Geometry check sheet. Reference: the model listing, model coordinates, mm. A direction names the side the tool comes from. Coordinates: 2 decimals unless noted, no trailing zeros. Write each loop counter-clockwise with the first axis right and the second up, starting at its lowest first coordinate (ties: lowest second). Pieces come first, ordered by that corner, then holes. Notation, with made-up numbers: (23.5, 49) -> (44.5, 49) arc R31 ccw to (44.5, 79) -> close; hole circle Ø8 at (52.25, -7). An arc over 180 degrees is marked (long way). Answer in a Markdown table with one row per item. Add a question column.
1. Cross-section at D-D on z = -3.81. Record the cut outline in (x, y).
2. Mould release check, pull along Z, two halves, no side actions. Record for faces 1 (the flat face through (4, 0, -73)), 2 (the flat face through (0, 2, -71)), 3 (the flat face through (63, 2, -143.764)): pulls with the +Z half, pulls with the -Z half, needs draft (parallel to the pull), parting line crosses it, or undercut.
3. Cross-section at C-C on x = 124.46. Record the cut outline in (y, z).
4. Scan lines: L1, parallel to X at y = 1.7, z = -3.81; L2, parallel to X at y = 1.5, z = -124; L3, parallel to X at y = 2.05, z = -139. Record each from-to range of solid material in increasing order. Write a range as from..to.
5. Set-up check for faces 4 (the flat face through (63, 2, 0)), 5 (the flat face through (63, 2, -128.524)), 6 (the flat face through (128.27, 2, -71)): record each of +Z, -Z, +X, -X, +Y, -Y from which the full face is reachable in a straight line by a thin tool's end or side.
6. Cross-section at A-A on z = -94.5. Record the cut outline in (x, y).
7. Cross-section at B-B on x = 20.5. Record the cut outline in (y, z).
8. Depth check by flat-ended pin: P1, Ø5, axis at x = 124.46, z = -139.954, coming from the -Y side; P2, Ø0.9, axis at x = 40.5, y = 1, coming from the -Z side; P3, Ø1.5, axis at y = 1, z = -45, coming from the +X side; P4, Ø0.9, axis at y = 2, z = -66, coming from the -X side. Enter the tip coordinate at first touch or a pass-through.
```python
from build123d import *

# Parameters (mm, degrees)
SKETCH1_W           = 128.27
SKETCH1_H           = 143.764
SKETCH1_W_2         = 97.79
SKETCH1_H_2         = 113.284
BOSS_EXTRUDE1_DEPTH = 3.048
SKETCH2_R           = 2.794
CUT_EXTRUDE1_DEPTH  = 3.302
SKETCH4_R           = 5.842
SKETCH4_R_2         = 2.794
BOSS_EXTRUDE2_DEPTH = 3.048


with BuildPart() as part:
    # Sketch1 → Boss-Extrude1 (new body)
    with BuildSketch(Plane(origin=(0, 0, 0), x_dir=(1, 0, 0), z_dir=(0, 1, 0))):
        with Locations((64.135, 71.882)):
            Rectangle(SKETCH1_W, SKETCH1_H)
        with Locations((64.135, 71.882)):
            Rectangle(SKETCH1_W_2, SKETCH1_H_2, mode=Mode.SUBTRACT)
    extrude(amount=BOSS_EXTRUDE1_DEPTH)

    # Sketch2 → Cut-Extrude1 (cut)
    with BuildSketch(Plane(origin=(0, 3.048, 0), x_dir=(1, 0, 0), z_dir=(0, 1, 0))):
        with Locations(Location((3.81, 139.954, 0), (0, 0, 270))):
            Circle(SKETCH2_R)
        with Locations(Location((124.46, 139.954, 0), (0, 0, 270))):
            Circle(SKETCH2_R)
        with Locations(Location((124.46, 3.81, 0), (0, 0, 270))):
            Circle(SKETCH2_R)
        with Locations(Location((3.81, 3.81, 0), (0, 0, 270))):
            Circle(SKETCH2_R)
    extrude(amount=-CUT_EXTRUDE1_DEPTH, mode=Mode.SUBTRACT)

    # Sketch4 → Boss-Extrude2 (add, through all)
    # profile 1 of 4: a face of its own
    with BuildSketch(Plane(origin=(0, 3.048, 0), x_dir=(1, 0, 0), z_dir=(0, 1, 0))):
        with Locations((3.81, 139.954)):
            Circle(SKETCH4_R)
        with Locations(Location((3.81, 139.954, 0), (0, 0, 270))):
            Circle(SKETCH4_R_2, mode=Mode.SUBTRACT)
    # profile 2 of 4: a face of its own
    with BuildSketch(Plane(origin=(0, 3.048, 0), x_dir=(1, 0, 0), z_dir=(0, 1, 0))):
        with Locations((124.46, 139.954)):
            Circle(SKETCH4_R)
        with Locations(Location((124.46, 139.954, 0), (0, 0, 270))):
            Circle(SKETCH4_R_2, mode=Mode.SUBTRACT)
    # profile 3 of 4: a face of its own
    with BuildSketch(Plane(origin=(0, 3.048, 0), x_dir=(1, 0, 0), z_dir=(0, 1, 0))):
        with Locations((124.46, 3.81)):
            Circle(SKETCH4_R)
        with Locations(Location((124.46, 3.81, 0), (0, 0, 270))):
            Circle(SKETCH4_R_2, mode=Mode.SUBTRACT)
    # profile 4 of 4: a face of its own
    with BuildSketch(Plane(origin=(0, 3.048, 0), x_dir=(1, 0, 0), z_dir=(0, 1, 0))):
        with Locations((3.81, 3.81)):
            Circle(SKETCH4_R)
        with Locations(Location((3.81, 3.81, 0), (0, 0, 270))):
            Circle(SKETCH4_R_2, mode=Mode.SUBTRACT)
    extrude(amount=-BOSS_EXTRUDE2_DEPTH)


solid = part.part
```
Results found:
| question | item | result |
|---|---|---|
| 1 | outline | (-2.03, 0) -> (1.02, 0) -> (1.02, 3.05) -> (-2.03, 3.05) -> close; (6.6, 0) -> (121.67, 0) -> (121.67, 3.05) -> (6.6, 3.05) -> close; (127.25, 0) -> (130.3, 0) -> (130.3, 3.05) -> (127.25, 3.05) -> close |
| 2 | face 1 | needs draft |
| 2 | face 2 | undercut |
| 2 | face 3 | pulls with the -Z half |
| 3 | outline | (0, -145.8) -> (3.05, -145.8) -> (3.05, -142.75) -> (0, -142.75) -> close; (0, -137.16) -> (3.05, -137.16) -> (3.05, -6.6) -> (0, -6.6) -> close; (0, -1.02) -> (3.05, -1.02) -> (3.05, 2.03) -> (0, 2.03) -> close |
| 4 | L1 | x = -2.03..1.02, 6.6..121.67, 127.25..130.3 |
| 4 | L2 | x = 0..15.24, 113.03..128.27 |
| 4 | L3 | x = -1.95..1.18, 6.44..121.83, 127.09..130.22 |
| 5 | face 4 | +Z, +Y, -Y |
| 5 | face 5 | +Y, -Y |
| 5 | face 6 | +X, +Y, -Y |
| 6 | outline | (0, 0) -> (15.24, 0) -> (15.24, 3.05) -> (0, 3.05) -> close; (113.03, 0) -> (128.27, 0) -> (128.27, 3.05) -> (113.03, 3.05) -> close |
| 7 | outline | (0, -143.76) -> (3.05, -143.76) -> (3.05, -128.52) -> (0, -128.52) -> close; (0, -15.24) -> (3.05, -15.24) -> (3.05, 0) -> (0, 0) -> close |
| 8 | P1 | passes through |
| 8 | P2 | stops at z = -143.76 |
| 8 | P3 | stops at x = 128.27 |
| 8 | P4 | stops at x = 0 |
